```python
from build123d import *

# Parameters (mm, degrees)
F0_W      = 110
F0_H      = 97
F0_R      = 2
F0_W_2    = 16
F0_H_2    = 46
F1_DEPTH  = 3
F2_W      = 22
F2_H      = 1.6
F3_DEPTH  = 1.6
F4_W      = 110
F4_H      = 97
F4_W_2    = 104
F4_H_2    = 91
F5_DEPTH  = 35
F6_W      = 25
F6_H      = 6
F7_DEPTH  = 8
F8_W      = 21
F8_H      = 3
F9_DEPTH  = 25
F11_DEPTH = 25
F12_W     = 21
F12_H     = 6
F13_DEPTH = 7
F15_DEPTH = 2
F16_R     = 1.207107
F18_DEPTH = 2
F19_R     = 1.2
F20_R     = 2
F21_DEPTH = 110.001


with BuildPart() as f1:
    # F0 (on Front) → F1 (new body)
    with BuildSketch(Plane.XZ):
        with Locations((67.24338, -70.311934)):
            Rectangle(F0_W, F0_H)
        with Locations((45.24338, -94.811934)):
            Circle(F0_R, mode=Mode.SUBTRACT)
        with Locations((74.24338, -94.811934)):
            Circle(F0_R, mode=Mode.SUBTRACT)
        with Locations((86.24338, -84.311934)):
            Rectangle(F0_W_2, F0_H_2, mode=Mode.SUBTRACT)
        with Locations((45.24338, -66.811934)):
            Circle(F0_R, mode=Mode.SUBTRACT)
    extrude(amount=F1_DEPTH)

    # F2 (on Front) → F3 (join)
    with BuildSketch(Plane.XZ):
        with Locations((67.24338, -25.611934)):
            Rectangle(F2_W, F2_H)
    extrude(amount=F3_DEPTH)

    # F4 (on face) → F5 (join)
    with BuildSketch(Plane.XZ.offset(3)):
        with Locations((67.24338, -70.311934)):
            Rectangle(F4_W, F4_H)
        with Locations((67.24338, -70.311934)):
            Rectangle(F4_W_2, F4_H_2, mode=Mode.SUBTRACT)
    extrude(amount=F5_DEPTH)

    # F6 (on face) → F7 (join)
    with BuildSketch(Plane.XY.offset(-21.811934)):
        with Locations((67.24338, -3)):
            Rectangle(F6_W, F6_H)
    extrude(amount=F7_DEPTH)

    # F8 (on face) → F9 (cut)
    with BuildSketch(Plane.XY.offset(-13.811934)):
        with Locations((67.24338, -3.3)):
            Rectangle(F8_W, F8_H)
    extrude(amount=-F9_DEPTH, mode=Mode.SUBTRACT)

    # F10 (on face) → F11 (cut)
    with BuildSketch(Plane(origin=(54.74338, 0, 0), x_dir=(0, -1, 0), z_dir=(-1, 0, 0))):
        with BuildLine():
            ThreePointArc((0, -15.811934), (0.585786, -14.397721), (2, -13.811934))
            Line((2, -13.811934), (0, -13.811934))
            Line((0, -13.811934), (0, -15.811934))
        make_face()
        with BuildLine():
            Line((6, -13.811934), (4, -13.811934))
            ThreePointArc((4, -13.811934), (5.414214, -14.397721), (6, -15.811934))
            Line((6, -15.811934), (6, -13.811934))
        make_face()
    extrude(amount=-F11_DEPTH, mode=Mode.SUBTRACT)

    # F12 (on face) → F13 (cut)
    with BuildSketch(Plane(origin=(0, 0, 0), x_dir=(-1, 0, 0), z_dir=(0, 1, 0))):
        with Locations((-67.24338, -16.811934)):
            Rectangle(F12_W, F12_H)
    extrude(amount=-F13_DEPTH, mode=Mode.SUBTRACT)

    # F14 (on face) → F15 (join)
    with BuildSketch(Plane(origin=(77.74338, 0, 0), x_dir=(0, -1, 0), z_dir=(-1, 0, 0))):
        with BuildLine():
            ThreePointArc((3, -13.961934), (1.621142, -17.290793), (4.95, -15.911934))
            ThreePointArc((4.95, -15.911934), (4.378858, -14.533076), (3, -13.961934))
        make_face()
    extrude(amount=F15_DEPTH)

    # F16
    f16_edges = [f1.edges().sort_by_distance(p)[0] for p in [
        (75.74338, -1.05, -15.911934),
    ]]
    fillet(f16_edges, radius=F16_R)

    # F17 (on face) → F18 (join)
    with BuildSketch(Plane.YZ.offset(56.74338)):
        with BuildLine():
            ThreePointArc((-3, -13.911934), (-4.414214, -17.326148), (-1, -15.911934))
            ThreePointArc((-1, -15.911934), (-1.585786, -14.497721), (-3, -13.911934))
        make_face()
    extrude(amount=F18_DEPTH)

    # F19
    f19_edges = [f1.edges().sort_by_distance(p)[0] for p in [
        (58.74338, -5, -15.911934),
    ]]
    fillet(f19_edges, radius=F19_R)

    # F20 (on face) → F21 (cut, through all)
    with BuildSketch(Plane.YZ.offset(122.24338)):
        with Locations((-28, -31.811934)):
            Circle(F20_R)
        with Locations((-28, -108.811934)):
            Circle(F20_R)
        with Locations((-28, -70.311934)):
            Circle(F20_R)
    extrude(amount=-F21_DEPTH, mode=Mode.SUBTRACT)


solid = f1.part
```
Input: part model. Units: mm. Frame: model coordinates. A direction names the side the tool comes from. Give positions to 0.01 mm unless a question says otherwise; leave off trailing zeros. Order: outer loops, then holes, each group sorted by start corner. A loop starts at its lowest first (then second) coordinate and runs counter-clockwise, first axis right, second up. Notation, with made-up numbers: (26, 77.25) - (66, 77.25) arc R9 cw to (66, 89.25) - close; hole circle Ø1 at (-1.5, 64). An arc over 180 degrees is marked (long way). Use a Markdown table: item, result.
(1) Section query B-B (y = -28). State how many separate pieces and enclosed holes the cut face has, then the cut area to 3 significant figures.
Computed values:
| item | result |
|---|---|
| separate pieces | 6 |
| enclosed holes | 0 |
| area | 1,130 mm2 |
(2) Section query D-D (z = -42). Output: boundary loops of the cut face in (x, y).
Computed values:
| item | result |
|---|---|
| outline | (12.24, -38) - (15.24, -38) - (15.24, -3) - (119.24, -3) - (119.24, -38) - (122.24, -38) - (122.24, 0) - (12.24, 0) - close |
(3) Pin query (flat end, axial travel): pin 1 (10 mm diameter, centred on x = 104, y = -22.5, fed in from +Z); pin 2 (10 mm diameter, centred on x = 104, z = -43.5, fed in from -Y); pin 3 (6.5 mm diameter, centred on y = -1.5, z = -17.5, fed in from -X); pin 4 (2.5 mm diameter, centred on x = 45.24, z = -66.81, fed in from -Y). Return the tip coordinate at first contact, or that it passes through.
Computed values:
| item | result |
|---|---|
| pin 1 | stops at z = -21.81 |
| pin 2 | stops at y = -3 |
| pin 3 | stops at x = 54.74 |
| pin 4 | passes through |
(4) Draft query along Z for faces 5 (the flat face through (66, -19, -118.812)), 6 (the flat face through (86, -1, -107.312)), 7 (the flat face through (66, 0, -67)). Return one class per face: released by +Z, released by -Z, zero draft, split by the parting line, or undercut.
Computed values:
| item | result |
|---|---|
| face 5 | released by -Z |
| face 6 | undercut |
| face 7 | zero draft |
(5) Section query C-C (x = 114). Output: boundary loops of the cut face in (y, z).
Computed values:
| item | result |
|---|---|
| outline | (-38, -118.81) - (0, -118.81) - (0, -21.81) - (-38, -21.81) - (-38, -24.81) - (-3, -24.81) - (-3, -115.81) - (-38, -115.81) - close |
(6) Section query A-A (z = -100). Output: boundary loops of the cut face in (x, y).
Computed values:
| item | result |
|---|---|
| outline | (12.24, -38) - (15.24, -38) - (15.24, -3) - (78.24, -3) - (78.24, 0) - (12.24, 0) - close; (94.24, -3) - (119.24, -3) - (119.24, -38) - (122.24, -38) - (122.24, 0) - (94.24, 0) - close |
(7) Line query: line 1 (Z direction, x = 120, y = -28); line 2 (X direction, y = -30, z = -57); line 3 (Z direction, x = 51, y = -16.5). Output: solid intervals per line, ascending. Write a range as from..to.
Computed values:
| item | result |
|---|---|
| line 1 | z = -118.81..-110.81, -106.81..-72.31, -68.31..-33.81, -29.81..-21.81 |
| line 2 | x = 12.24..15.24, 119.24..122.24 |
| line 3 | z = -118.81..-115.81, -24.81..-21.81 |
(8) Access query for faces 1 (the flat face through (119.243, -20, -71)), 2 (the flat face through (56.743, -3, -24)), 3 (the flat face through (79.743, -3, -18)), 4 (the flat face through (94.243, -1, -85)). Directions: +Z, -Z, +X, -X, +Y, -Y. A direction counts if a zero-diameter tool reaches every point of the face in a straight line with its end or side. Return the directions, or none.
Computed values:
| item | result |
|---|---|
| face 1 | -Y |
| face 2 | none |
| face 3 | +Z, +X, +Y, -Y |
| face 4 | +Y, -Y |
